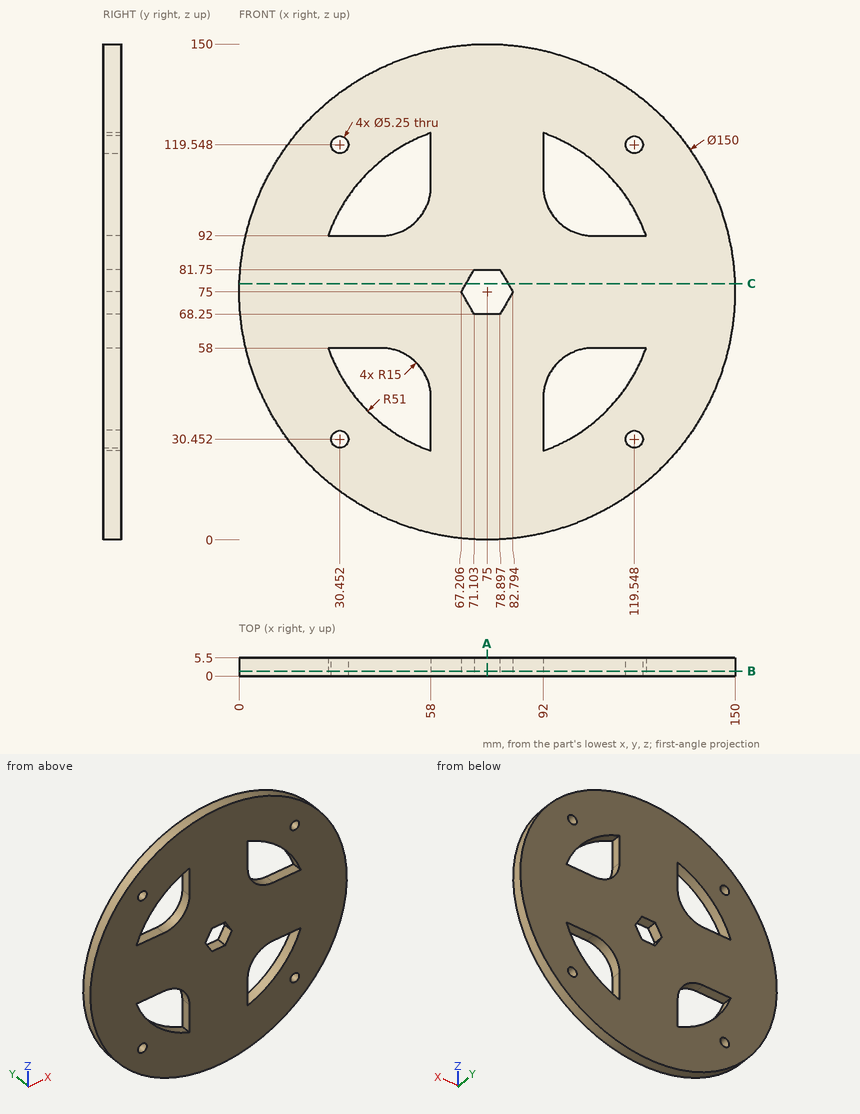
Could you check a few things on this drawing? It's one solid part, dimensions in mm from its lowest x, y, z. Give positions to 0.01 mm unless a question says otherwise; leave off trailing zeros. Write each loop counter-clockwise with the first axis right and the second up, starting at its lowest first coordinate (ties: lowest second). Pieces come first, ordered by that corner, then holes. Notation, with made-up numbers: M -8,40 L 15,40 A29 ccw 15,76 Z; hole C 56.5,75.25 d11. An arc over 180 degrees is marked long. Put each result on its own line as item: value. Start each with the question number.
Item 1: Will these pins go through, and if not, where does the flat tip stop? pin 1 (6 mm diameter, centred on x = 118, z = 77.5, fed in from -Y); pin 2 (3 mm diameter, centred on x = 115, y = 3, fed in from -Z); pin 3 (3 mm diameter, centred on x = 127.5, y = 2.5, fed in from -Z); pin 4 (3 mm diameter, centred on y = 3, z = 118.5, fed in from +X).
Item 2: If we section it at A-A, the plane x = 75: Write out the boundary of the cut face in (y, z).
Item 3: If we section it at C-C, the plane z = 77.5: Write out the boundary of the cut face in (x, y).
Item 4: I need wall thicknesses on L1, parallel to X at y = 4.05, z = 95.5 (1 decimal); L2, parallel to Z at x = 112.5, y = 1.75 (1 decimal); L3, parallel to Z at x = 113.5, y = 3.75 (1 decimal). Which ranges of each line are inside material? Lowest first, please. Write a range as from..to.
Item 5: If we section it at B-B, the plane y = 1.45: Count the separate pieces of the cut face and the enclosed holes in it, then the cut area to 3 significant figures.
Values:
1. pin 1: y = 0
1. pin 2: z = 10.64
1. pin 3: z = 20.01
1. pin 4: x = 137.14
2. outline: M 0,0 L 5.5,0 L 5.5,68.25 L 0,68.25 Z; M 0,81.75 L 5.5,81.75 L 5.5,150 L 0,150 Z
3. outline: M 0.04,0 L 68.65,0 L 68.65,5.5 L 0.04,5.5 Z; M 81.35,0 L 149.96,0 L 149.96,5.5 L 81.35,5.5 Z
4. L1: 2.9..28.3, 52.6..97.4, 121.7..147.1
4. L2: 10..40.4, 58..92, 109.6..140
4. L3: 10.6..41.6, 58..92, 108.4..139.4
5. separate pieces: 1
5. enclosed holes: 9
5. area: 15,100 mm²
